```python
from build123d import *

# Parameters (mm, degrees)
SKETCH1_W           = 15
SKETCH1_H           = 9
BOSS_EXTRUDE1_DEPTH = 5
SKETCH2_W           = 7.408175253
SKETCH2_H           = 9
SKETCH2_W_2         = 8.292733492
BOSS_EXTRUDE2_DEPTH = 5


with BuildPart() as part:
    # Sketch1 → Boss-Extrude1 (new body)
    with BuildSketch(Plane.XY):
        Rectangle(SKETCH1_W, SKETCH1_H)
    extrude(amount=BOSS_EXTRUDE1_DEPTH)

    # Sketch2 → Boss-Extrude2 (add)
    with BuildSketch(Plane.XY):
        with Locations((-8.00051336, 0)):
            Rectangle(SKETCH2_W, SKETCH2_H)
        with Locations((6.768450098, 0)):
            Rectangle(SKETCH2_W_2, SKETCH2_H)
    extrude(amount=-BOSS_EXTRUDE2_DEPTH)


solid = part.part
```
Input: part model. Units: mm. Frame: model coordinates. A direction names the side the tool comes from. Coordinates: 2 decimals unless noted, no trailing zeros. Loops run counter-clockwise (first coordinate to the right, second up) from the corner with the lowest first, then second, coordinate; pieces in that order, holes last.
Q1. Section A-A, the plane z = -2.25. Return the cut outline in (x, y), and give its area (3 significant figures).
Results are:
outline: (-11.7, -4.5) - (-4.3, -4.5) - (-4.3, 4.5) - (-11.7, 4.5) - close; (2.62, -4.5) - (10.91, -4.5) - (10.91, 4.5) - (2.62, 4.5) - close
area: 141 mm2
Q2. Contact query for flat-ended pins moving along their axis: pin 1 (1.5 mm diameter, centred on y = -1.5, z = 2.5, fed in from +X); pin 2 (3.5 mm diameter, centred on x = -10, y = -1, fed in from +Z); pin 3 (3.5 mm diameter, centred on x = 0, y = -0.5, fed in from -Z). Output: stop coordinate, or through.
Results are:
pin 1: stops at x = 7.5
pin 2: stops at z = 0
pin 3: stops at z = 0
Q3. Mould query, pull axis X, two halves, no side actions, for faces 1 (the flat face through (0, 0, 5)), 2 (the flat face through (-11.705, 0, -2)), 3 (the flat face through (2.622, 0, -2)), 4 (the flat face through (10.915, 0, -2)). Classes: +X half, -X half, draft (parallel to the pull), parting line (faces both ways), or undercut.
Results are:
face 1: draft
face 2: -X half
face 3: undercut
face 4: +X half
Q4. Section B-B, the plane y = 3. Return the cut outline in (x, z).
Results are:
outline: (-11.7, -5) - (-4.3, -5) - (-4.3, 0) - (2.62, 0) - (2.62, -5) - (10.91, -5) - (10.91, 0) - (7.5, 0) - (7.5, 5) - (-7.5, 5) - (-7.5, 0) - (-11.7, 0) - close
Q5. Line query: line 1 along X through (y, z) = (0.25, -0.25); line 2 along Z through (x, y) = (-3.5, 1.5); line 3 along Z through (x, y) = (9.25, 4). Output: solid intervals per line, ascending.
Results are:
line 1: x = -11.7 to -4.3, 2.62 to 10.91
line 2: z = 0 to 5
line 3: z = -5 to 0
Q6. Section C-C, the plane x = -0.25. Return the cut outline in (y, z).
Results are:
outline: (-4.5, 0) - (4.5, 0) - (4.5, 5) - (-4.5, 5) - close
Q7. Section D-D, the plane z = 4.25. Return the cut outline in (x, y).
Results are:
outline: (-7.5, -4.5) - (7.5, -4.5) - (7.5, 4.5) - (-7.5, 4.5) - close
Q8. Set-up query: faces 5 (the flat face through (-10, 0, 0)), 6 (the flat face through (-1, 0, 0)), 7 (the flat face through (9, 0, 0)). Return all of +Z, -Z, +X, -X, +Y, -Y with unobstructed straight access to the full face (end or side cutting, diameter ignored); none if empty.
Results are:
face 5: +Z, -X, +Y, -Y
face 6: -Z, +Y, -Y
face 7: +Z, +X, +Y, -Y
